from build123d import *

# Parameters (mm, degrees)
SKETCH1_W           = 12.7
SKETCH1_H           = 125.73
BOSS_EXTRUDE1_DEPTH = 10.16
SKETCH4_W           = 7.874
SKETCH4_H           = 7.874
CUT_EXTRUDE2_DEPTH  = 6.35
SKETCH6_W           = 7.874
SKETCH6_H           = 7.874
CUT_EXTRUDE4_DEPTH  = 6.35
SKETCH8_W           = 7.874
SKETCH8_H           = 7.874
CUT_EXTRUDE5_DEPTH  = 6.35


with BuildPart() as part:
    # Sketch1 → Boss-Extrude1 (new body)
    with BuildSketch(Plane.XY):
        with Locations((0, 75.565)):
            Rectangle(SKETCH1_W, SKETCH1_H)
    extrude(amount=BOSS_EXTRUDE1_DEPTH)

    # Sketch4 → Cut-Extrude2 (cut)
    with BuildSketch(Plane(origin=(0, 138.43, 0), x_dir=(1, 0, 0), z_dir=(0, 1, 0))):
        with Locations((0, -5.08)):
            Rectangle(SKETCH4_W, SKETCH4_H)
    extrude(amount=-CUT_EXTRUDE2_DEPTH, mode=Mode.SUBTRACT)

    # Sketch6 → Cut-Extrude4 (cut)
    with BuildSketch(Plane.XY.offset(10.16)):
        with Locations((0, 25.4)):
            Rectangle(SKETCH6_W, SKETCH6_H)
    extrude(amount=-CUT_EXTRUDE4_DEPTH, mode=Mode.SUBTRACT)

    # Sketch8 → Cut-Extrude5 (cut)
    with BuildSketch(Plane.XZ.offset(-12.7)):
        with Locations((0, 5.08)):
            Rectangle(SKETCH8_W, SKETCH8_H)
    extrude(amount=-CUT_EXTRUDE5_DEPTH, mode=Mode.SUBTRACT)


solid = part.part
Geometry check sheet. Reference: the model listing, model coordinates, mm. A direction names the side the tool comes from. Give positions to 0.01 mm unless a question says otherwise; leave off trailing zeros. Loops run counter-clockwise (first coordinate to the right, second up) from the corner with the lowest first, then second, coordinate; pieces in that order, holes last. Notation, with made-up numbers: M -26,60.5 L -9,60.5 A23 ccw -9,72.5 Z; hole C 26,-37 d6. An arc over 180 degrees is marked long. Answer as a JSON object with one key per item and string values. Group by question number.
Item 1: Access from +Z, -Z, +X, -X, +Y, -Y to the whole of each face (thin tool, end or side, straight path). Record for faces 1 (the flat face through (6.35, 75, 5)), 2 (the flat face through (0, 29.337, 7)), 3 (the flat face through (0, 76, 0)), 4 (the flat face through (0, 16, 9.017)), 5 (the flat face through (0, 135, 1.143)).
Item 2: Sectioned sample at D-D on y = 27. Record the boundary of the cut face in (x, z), plus the area to 3 significant figures.
Item 3: Sectioned sample at C-C on z = 2.75. Record the boundary of the cut face in (x, y), plus the area to 3 significant figures.
Item 4: Mould release check, pull along Y, two halves, no side actions. Record for faces 6 (the flat face through (4.1, 138.43, 5)), 7 (the flat face through (4.1, 12.7, 5)), 8 (the flat face through (3.937, 25, 7)), 9 (the flat face through (0, 76, 10.16)): pulls with the +Y half, pulls with the -Y half, needs draft (parallel to the pull), parting line crosses it, or undercut.
Item 5: Material ranges on L1, parallel to Y at x = 2.5, z = 6.25; L2, parallel to Y at x = -1, z = 9.25; L3, parallel to Z at x = 3.5, y = 133, recorded low to high.
Item 6: Sectioned sample at B-B on x = 0. Record the boundary of the cut face in (y, z), plus the area to 3 significant figures.
Item 7: Sectioned sample at A-A on z = 7.75. Record the boundary of the cut face in (x, y).
Item 8: Gauge pin test, flat end, axial feed: pin 1 (4 mm diameter, centred on x = 1, z = 3.5, fed in from -Y). Record the tip position at first contact, or that the pin passes through.
Findings below:
{
 "1": {"face 1": "+Z, -Z, +X, +Y, -Y", "face 2": "+Z", "face 3": "-Z, +X, -X, +Y, -Y", "face 4": "-Y", "face 5": "+Y"},
 "2": {"outline": "M -6.35,0 L 6.35,0 L 6.35,10.16 L 3.94,10.16 L 3.94,3.81 L -3.94,3.81 L -3.94,10.16 L -6.35,10.16 Z", "area": "79.0 mm2"},
 "3": {"outline": "M -6.35,12.7 L -3.94,12.7 L -3.94,19.05 L 3.94,19.05 L 3.94,12.7 L 6.35,12.7 L 6.35,138.43 L 3.94,138.43 L 3.94,132.08 L -3.94,132.08 L -3.94,138.43 L -6.35,138.43 Z", "area": "1,500 mm2"},
 "4": {"face 6": "pulls with the +Y half", "face 7": "pulls with the -Y half", "face 8": "undercut", "face 9": "needs draft"},
 "5": {"L1": "19.05 to 21.46, 29.34 to 132.08", "L2": "12.7 to 21.46, 29.34 to 138.43", "L3": "0 to 1.14, 9.02 to 10.16"},
 "6": {"outline": "M 12.7,0 L 138.43,0 L 138.43,1.14 L 132.08,1.14 L 132.08,9.02 L 138.43,9.02 L 138.43,10.16 L 29.34,10.16 L 29.34,3.81 L 21.46,3.81 L 21.46,10.16 L 12.7,10.16 L 12.7,9.02 L 19.05,9.02 L 19.05,1.14 L 12.7,1.14 Z", "area": "1,130 mm2"},
 "7": {"outline": "M -6.35,12.7 L -3.94,12.7 L -3.94,19.05 L 3.94,19.05 L 3.94,12.7 L 6.35,12.7 L 6.35,138.43 L 3.94,138.43 L 3.94,132.08 L -3.94,132.08 L -3.94,138.43 L -6.35,138.43 Z; hole M -3.94,21.46 L 3.94,21.46 L 3.94,29.34 L -3.94,29.34 Z"},
 "8": {"pin 1": "y = 19.05"}
}
